Autodesk Inventor part; units mm, degrees
ref_plane "YZ Plane" through (0, 0, 0) normal (1, 0, 0) x (0, 1, 0)
ref_plane "XZ Plane" through (0, 0, 0) normal (0, 1, 0) x (-1, 0, 0)
ref_plane "XY Plane" through (0, 0, 0) normal (0, 0, 1) x (1, 0, 0)
sketch "Sketch1" plane through (0, 0, 0) normal (0, 1, 0) x (-1, 0, 0)
  line L0 (0, 0) -> (30, 0)
  line L1 (0, 0) -> (0, -37)
  line L2 (0, -37) -> (30, -37)
  line L3 (30, 0) -> (30, 3)
  line L4 (30, 3) -> (-5, 3)
  line L5 (-5, 3) -> (-5, -40)
  line L6 (-5, -40) -> (30, -40)
  line L7 (30, -40) -> (30, -37)
  dimension "d0" = 30
  dimension "d1" = 37
  dimension "d2" = 30
  dimension "d3" = 90
  dimension "d4" = 3
  dimension "d5" = 35
  dimension "d6" = 43
extrude "Extrusion1" add sketch "Sketch1" along normal blind 30
fillet "Fillet1" radius 2 4 edges at (5, 15, 3) (5, 15, -40) (0, 15, -37) (0, 15, 0)
sketch "Sketch2" plane through (5, 0, 1) normal (1, 0, 0) x (0, 0, -1)
  line L0 (39, 30) -> (39, 0)
  line L1 (0, 30) -> (39, 30)
  line L2 (0, 0) -> (0, 30)
  line L3 (0, 0) -> (39, 0)
  circle A0 centre (19.5, 15) radius 5
  circle A1 centre (19.5, 15) radius 7
  point P0 (1, 0)
  dimension "d10" = 10
  dimension "d11" = 14
extrude "Extrusion2" add sketch "Sketch2" along normal blind 30 contours A1
fillet "Fillet2" radius 2 1 edges at (5, 15, -11.5)
fillet "Fillet3" radius 15 4 edges at (-30, 30, 1.5) (-30, 0, 1.5) (-30, 30, -38.5) (-30, 0, -38.5)
sketch "Sketch3" plane through (3, 0, 3) normal (0, 0, 1) x (1, 0, 0)
  arc A0 (-18, 30) -> (-18, 0) centre (-18, 15) ccw
  line L0 (-18, 0) -> (0, 0)
  line L1 (0, 30) -> (0, 0)
  line L2 (-18, 30) -> (0, 30)
  circle A1 centre (-21.5, 15) radius 11
  point P0 (-3, 0)
  point P1 (-29.5, 15)
  point P2 (-21.5, 23)
  point P3 (-13.5, 15)
  point P4 (-21.5, 7)
  dimension "d16" = 22
  dimension "d18" = 8
  dimension "d19" = 8
  dimension "d20" = 8
  dimension "d21" = 8
hole "Hole1" at (-18.5, 15, 3) at (-26.5, 15, 3) at (-18.5, 23, 3) at (-10.5, 15, 3) at (-18.5, 7, 3) direction (0, 0, -1) diameter 2 depth 8 tip angle 118
sketch "Sketch4" plane through (3, 0, -40) normal (0, 0, -1) x (-1, 0, 0)
  circle A0 centre (13.5, 15) radius 1
  circle A1 centre (29.5, 15) radius 1
  circle A2 centre (21.5, 15) radius 1
  circle A3 centre (21.5, 23) radius 1
  circle A4 centre (21.5, 7) radius 1
  arc A5 (18, 0) -> (18, 30) centre (18, 15) ccw
  line L0 (5, 30) -> (18, 30)
  line L1 (5, 0) -> (5, 30)
  line L2 (5, 0) -> (18, 0)
  point P0 (3, 0)
hole "Hole2" at (-18.5, 15, -40) direction (0, 0, 1) diameter 4 end through all
properties part number "Pen"
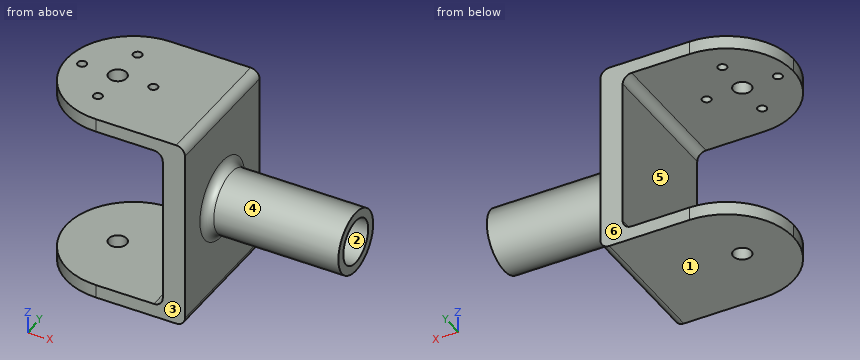
Geometry: final body of the model. Coordinates: model frame, mm. Face numbers are marked on the shaded views. A direction names the side the tool comes from. Coordinates: 2 decimals unless noted, no trailing zeros. Loops run counter-clockwise (first coordinate to the right, second up) from the corner with the lowest first, then second, coordinate; pieces in that order, holes last. Notation, with made-up numbers: M 59,-11 L 111,-11 A18 cw 111,1 Z; hole C 2,-22.75 d7. An arc over 180 degrees is marked long. One line per item, written item: value. Start each with the question number.
1) Material intervals for L1, parallel to Z at x = -19.5, y = 18.75; L2, parallel to Y at x = -18, z = 1; L3, parallel to Y at x = -18.5, z = 1.5, sorted ascending. Write a range as from..to.
2) Draft query along Z for the marked faces 1, 2 and 3. Return one class per face: released by +Z, released by -Z, zero draft, split by the parting line, or undercut.
3) Pin query (flat end, axial travel): P1, Ø15, axis at y = 10.5, z = -11.5, coming from the -X side; P2, Ø1.5, axis at y = 6, z = -32, coming from the +X side; P3, Ø2.5, axis at x = -18.5, y = 15, coming from the -Z side; P4, Ø6, axis at x = 28, y = 14, coming from the -Z side. Return the tip coordinate at first contact, or that it passes through.
4) Cut plane D-D (y = 2.75). Return loops of the section in (x, z).
5) Cut plane A-A (x = -10.5). Return loops of the section in (y, z), then the cut area to 3 significant figures.
6) Reachability of the marked faces 4, 5 and 6 from +Z, -Z, +X, -X, +Y, -Y: full face, straight path, thin tool, end or side. Return the list, or none.
7) Cut plane B-B (z = -18.5). Return loops of the section in (x, y).
8) Cut plane C-C (x = -18.5). Return loops of the section in (y, z), then the cut area to 3 significant figures.
Evaluation:
1. L1: -40..-37, 0..3
1. L2: 0.3..6.13, 7.87..13.06, 16.94..22.13, 23.87..29.7
1. L3: 0.41..6, 8..13, 17..22, 24..29.59
2. face 1: released by -Z
2. face 2: undercut
2. face 3: zero draft
3. P1: x = 0
3. P2: x = 5
3. P3: through
3. P4: z = -25.5
4. outline: M -23.66,-40 L 3,-40 A2 ccw 5,-38 L 5,1 A2 ccw 3,3 L -23.66,3 L -23.66,0 L -2,0 A2 cw 0,-2 L 0,-35 A2 cw -2,-37 L -23.66,-37 Z
5. outline: M 0,-40 L 30,-40 L 30,-37 L 0,-37 Z; M 0,0 L 14,0 L 14,3 L 0,3 Z; M 16,0 L 30,0 L 30,3 L 16,3 Z
5. area: 174 mm^2
6. face 4: +X
6. face 5: -X, +Y, -Y
6. face 6: +Z, -Z, +X, -X, +Y
7. outline: M 0,0 L 5,0 L 5,6 A2 cw 7,8 L 35,8 L 35,10 L 5,10 L 5,20 L 35,20 L 35,22 L 7,22 A2 cw 5,24 L 5,30 L 0,30 Z
8. outline: M 0.41,-40 L 13,-40 L 13,-37 L 0.41,-37 Z; M 0.41,0 L 6,0 L 6,3 L 0.41,3 Z; M 8,0 L 13,0 L 13,3 L 8,3 Z; M 17,-40 L 29.59,-40 L 29.59,-37 L 17,-37 Z; M 17,0 L 22,0 L 22,3 L 17,3 Z; M 24,0 L 29.59,0 L 29.59,3 L 24,3 Z
8. area: 139 mm^2
